Model file for the job. Use its own axes, mm. Give positions to 0.01 mm unless a question says otherwise; leave off trailing zeros. Write each loop counter-clockwise with the first axis right and the second up, starting at its lowest first coordinate (ties: lowest second). Pieces come first, ordered by that corner, then holes.
```python
from build123d import *

# Parameters (mm, degrees)
SKETCH1_W           = 120
SKETCH1_H           = 120
SKETCH1_R           = 2.375
BOSS_EXTRUDE1_DEPTH = 4.7625


with BuildPart() as part:
    # Sketch1 → Boss-Extrude1 (new body)
    with BuildSketch(Plane(origin=(0, 0, 0), x_dir=(1, 0, 0), z_dir=(0, 1, 0))):
        with Locations((60, 60)):
            Rectangle(SKETCH1_W, SKETCH1_H)
        with Locations((30, 90)):
            Circle(SKETCH1_R, mode=Mode.SUBTRACT)
        with Locations((45, 90)):
            Circle(SKETCH1_R, mode=Mode.SUBTRACT)
        with Locations((60, 90)):
            Circle(SKETCH1_R, mode=Mode.SUBTRACT)
        with Locations((75, 90)):
            Circle(SKETCH1_R, mode=Mode.SUBTRACT)
        with Locations((90, 90)):
            Circle(SKETCH1_R, mode=Mode.SUBTRACT)
        with Locations((97.5, 60)):
            Circle(SKETCH1_R, mode=Mode.SUBTRACT)
        with Locations((82.5, 60)):
            Circle(SKETCH1_R, mode=Mode.SUBTRACT)
        with Locations((67.5, 60)):
            Circle(SKETCH1_R, mode=Mode.SUBTRACT)
        with Locations((52.5, 60)):
            Circle(SKETCH1_R, mode=Mode.SUBTRACT)
        with Locations((37.5, 60)):
            Circle(SKETCH1_R, mode=Mode.SUBTRACT)
        with Locations((22.5, 30)):
            Circle(SKETCH1_R, mode=Mode.SUBTRACT)
        with Locations((37.5, 30)):
            Circle(SKETCH1_R, mode=Mode.SUBTRACT)
        with Locations((52.5, 30)):
            Circle(SKETCH1_R, mode=Mode.SUBTRACT)
        with Locations((67.5, 30)):
            Circle(SKETCH1_R, mode=Mode.SUBTRACT)
        with Locations((82.5, 30)):
            Circle(SKETCH1_R, mode=Mode.SUBTRACT)
        with Locations((97.5, 30)):
            Circle(SKETCH1_R, mode=Mode.SUBTRACT)
        with Locations((22.5, 60)):
            Circle(SKETCH1_R, mode=Mode.SUBTRACT)
    extrude(amount=BOSS_EXTRUDE1_DEPTH)


solid = part.part
```
1. Pull direction X, two halves, no side cores. Call faces 1 (the cylindrical face through (89.49, 2.35, -87.68)), 2 (the flat face through (59, 2, 0)), 3 (the flat face through (120, 2, -59)): +X half, -X half, draft (parallel to the pull), parting line (faces both ways), or undercut.
Calculated:
face 1: undercut
face 2: draft
face 3: +X half
2. Slice it at C-C, the plane x = 75. Write the cut outline in (y, z) (1 decimal).
Calculated:
outline: (0, -120) - (4.8, -120) - (4.8, -92.4) - (0, -92.4) - close; (0, -87.6) - (4.8, -87.6) - (4.8, 0) - (0, 0) - close
3. Probe probe 1 along Z at (x, y) = (22.5, 2.95) (3 decimals); probe 2 along X at (y, z) = (3.5, -90) (3 decimals); probe 3 along X at (y, z) = (3.95, -88). List the from-to ranges inside material, lowest first.
Calculated:
probe 1: z = -120 to -62.375, -57.625 to -32.375, -27.625 to 0
probe 2: x = 0 to 27.625, 32.375 to 42.625, 47.375 to 57.625, 62.375 to 72.625, 77.375 to 87.625, 92.375 to 120
probe 3: x = 0 to 28.72, 31.28 to 43.72, 46.28 to 58.72, 61.28 to 73.72, 76.28 to 88.72, 91.28 to 120
4. Slice it at A-A, the plane y = 1.8. State how many separate pieces and enclosed holes the cut face has, and give its area (3 significant figures).
Calculated:
separate pieces: 1
enclosed holes: 17
area: 14,100 mm2
5. Slice it at B-B, the plane x = 22.5. Write the cut outline in (y, z) (1 decimal).
Calculated:
outline: (0, -120) - (4.8, -120) - (4.8, -62.4) - (0, -62.4) - close; (0, -57.6) - (4.8, -57.6) - (4.8, -32.4) - (0, -32.4) - close; (0, -27.6) - (4.8, -27.6) - (4.8, 0) - (0, 0) - close
